For this review, take the finished solid that the model builds, in its own axes (mm). A direction names the side the tool comes from. Round coordinates to 2 decimals unless told otherwise and drop trailing zeros. Order: outer loops, then holes, each group sorted by start corner. A loop starts at its lowest first (then second) coordinate and runs counter-clockwise, first axis right, second up. Notation, with made-up numbers: M 42.5,24.5 L 93.5,24.5 A25 cw 93.5,50.5 Z; hole C 71.5,50 d4. An arc over 180 degrees is marked long. Answer as a JSON object with one key per item and string values.
from build123d import *

# Parameters (mm, degrees)
BOSS_EXTRUDE1_DEPTH = 1.524


with BuildPart() as part:
    # Sketch1 → Boss-Extrude1 (new body)
    with BuildSketch(Plane.XY):
        with BuildLine():
            Line((26.703585716, 0), (26.703585716, -1.524))
            Line((26.703585716, -1.524), (28.227585716, -1.524))
            Line((28.227585716, -1.524), (28.227585716, 0))
            Line((28.227585716, 0), (30.562754439, 1.639658569))
            Line((30.562754439, 1.639658569), (31.438516966, 0.39241521))
            Line((31.438516966, 0.39241521), (32.685760325, 1.268177737))
            Line((32.685760325, 1.268177737), (31.809997798, 2.515421096))
            Line((31.809997798, 2.515421096), (33.306965818, 3.566529915))
            ThreePointArc((33.306965818, 3.566529915), (32.151803022, 4.293127988), (30.792442306, 4.172777296))
            Line((30.792442306, 4.172777296), (24.84965689, 0))
            Line((24.84965689, 0), (26.703585716, 0))
        make_face()
    extrude(amount=BOSS_EXTRUDE1_DEPTH)


solid = part.part
1) Mouldability with a two-part tool opening along X and no side actions: class faces 5 (the flat face through (30.995, 1.025, 0.751)), 6 (the flat face through (27.863, 2.116, 0.751)), 7 (the flat face through (28.228, -1, 1)), 8 (the flat face through (26, 0, 1)) as +X half, -X half, draft (parallel to the pull), parting line (faces both ways), or undercut.
Geometry check:
{"face 5": "undercut", "face 6": "-X half", "face 7": "+X half", "face 8": "draft"}
2) Add section C-C on y = 1.4. State the section outline as (x, z) points.
Geometry check:
{"outline": "M 26.84,0 L 30.22,0 L 30.22,1.52 L 26.84,1.52 Z; M 30.73,0 L 32.59,0 L 32.59,1.52 L 30.73,1.52 Z"}
3) Add section A-A on x = 32. State the section outline as (y, z) points, and give its area (3 significant figures).
Geometry check:
{"outline": "M 0.79,0 L 2.24,0 L 2.24,1.52 L 0.79,1.52 Z; M 2.65,0 L 4.32,0 L 4.32,1.52 L 2.65,1.52 Z", "area": "4.78 mm²"}
4) Insertion check: P1, Ø0.8, axis at y = -1, z = 1, coming from the +X side; P2, Ø0.5, axis at x = 25.5, z = 0.5, coming from the -Y side. Each pin has a flat end and moves straight along its axis. Give the tip position at first contact, or say it passes through.
Geometry check:
{"P1": "stops at x = 28.23", "P2": "stops at y = 0"}
5) Machinability: for faces 1 (the flat face through (32.5, 3, 0.8)), 2 (the flat face through (32.05, 0.82, 0.75)), 3 (the flat face through (29.38, 0.81, 0.75)), 4 (the flat face through (26.704, -1, 1)), which of the approach directions +Z, -Z, +X, -X, +Y, -Y give a long, thin tool a straight path to every point of the face, cutting with its end or side? Answer none if there is none.
Geometry check:
{"face 1": "+Z, -Z, +X", "face 2": "+Z, -Z, +X, -Y", "face 3": "+Z, -Z, -Y", "face 4": "+Z, -Z, -X, -Y"}
6) For L1, parallel to X at y = -0.9, z = 0.5; L2, parallel to Y at x = 32.5, z = 0.6; L3, parallel to Y at x = 32, z = 0.4, list the stretches that pass through material, from the lowest coordinate up.
Geometry check:
{"L1": "x = 26.7 to 28.23", "L2": "y = 1.14 to 1.53, 3 to 4.18", "L3": "y = 0.79 to 2.24, 2.65 to 4.32"}
7) Add section D-D on y = -0.35. State the section outline as (x, z) points.
Geometry check:
{"outline": "M 26.7,0 L 28.23,0 L 28.23,1.52 L 26.7,1.52 Z"}
8) Add section B-B on z = 0.65. State the section outline as (x, y) points.
Geometry check:
{"outline": "M 24.85,0 L 26.7,0 L 26.7,-1.52 L 28.23,-1.52 L 28.23,0 L 30.56,1.64 L 31.44,0.39 L 32.69,1.27 L 31.81,2.52 L 33.31,3.57 A2.14 ccw 30.79,4.17 Z"}
